Could you check a few things on this model? Use its own coordinates, in mm. Face numbers are marked on the shaded views. A direction names the side the tool comes from. Give positions to 0.01 mm unless a question says otherwise; leave off trailing zeros. Write each loop counter-clockwise with the first axis right and the second up, starting at its lowest first coordinate (ties: lowest second). Pieces come first, ordered by that corner, then holes. Notation, with made-up numbers: (6.5, 55.25) -> (34.5, 55.25) arc R26 ccw to (34.5, 73.25) -> close; hole circle Ø3 at (53, 21.5). An arc over 180 degrees is marked (long way). One line per question, with ' | ' between items.
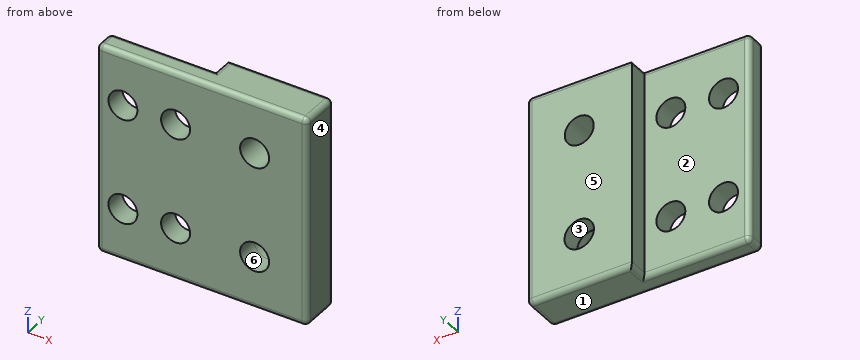
Autodesk Inventor part; units mm, degrees
ref_plane "YZ Plane" through (0, 0, 0) normal (1, 0, 0) x (0, 1, 0)
ref_plane "XZ Plane" through (0, 0, 0) normal (0, 1, 0) x (-1, 0, 0)
ref_plane "XY Plane" through (0, 0, 0) normal (0, 0, 1) x (1, 0, 0)
sketch "Sketch1" plane through (0, 0, 0) normal (0, 1, 0) x (-1, 0, 0)
  line L0 (17.7143, 25.1429) -> (-22.2857, 25.1429)
  line L1 (-22.2857, 25.1429) -> (-22.2857, -14.8571)
  line L2 (-22.2857, -14.8571) -> (17.7143, -14.8571)
  line L3 (17.7143, -14.8571) -> (17.7143, 25.1429)
  circle A0 centre (12.7143, 15.1429) radius 2.75
  circle A1 centre (12.7143, -4.8571) radius 2.75
  circle A2 centre (2.7143, -4.8571) radius 2.75
  circle A3 centre (2.7143, 15.1429) radius 2.75
  circle A4 centre (-12.2857, 15.1429) radius 2.75
  circle A5 centre (-12.2857, -4.8571) radius 2.75
  point P0 (0, 0)
  dimension "d1" = 40
  dimension "d2" = 5.5
  dimension "d3" = 5.5
  dimension "d4" = 5.5
  dimension "d5" = 5.5
  dimension "d6" = 5.5
  dimension "d7" = 5.5
  dimension "d9" = 10
  dimension "d12" = 20
  dimension "d13" = 10
  dimension "d17" = 5
  dimension "d28" = 10
  dimension "d32" = 15
extrude "Extrusion1" add sketch "Sketch1" along normal blind 4
sketch "Sketch2" plane through (0, 4, 0) normal (0, 1, 0) x (1, 0, 0)
  line L0 (22.2857, -25.1429) -> (22.2857, 14.8571)
  line L1 (22.2857, 14.8571) -> (2.2857, 14.8571)
  line L2 (2.2857, 14.8571) -> (2.2857, -25.1429)
  line L3 (2.2857, -25.1429) -> (22.2857, -25.1429)
  line L4 (22.2857, -25.1429) -> (22.2857, 14.8571)
  point P0 (0, 0)
  dimension "d30" = 20
  dimension "d31" = 40
extrude "Extrusion2" add sketch "Sketch2" along normal blind 3.7
sketch "Sketch3" plane through (12.2857, 4, -4.8571) normal (0, -1, 0) x (1, 0, 0)
  circle A0 centre (0, 0) radius 2.7975
  circle A1 centre (0, 20) radius 2.75
  line L0 (10, -10) -> (-30, -10)
  line L1 (10, 30) -> (10, -10)
  point P0 (-12.2857, 4.8571)
  dimension "d21" = 20
  dimension "d22" = 5.5
  dimension "d23" = 10
  dimension "d24" = 10
extrude "Extrusion3" cut sketch "Sketch3" against normal blind 3.7
fillet "Fillet2" radius 1 16 edges at (2.2857, 0, 25.1429) (-7.7143, 4, 25.1429) (12.2857, 7.7, 25.1429) (22.2857, 3.85, 25.1429) (22.2857, 7.7, 5.1429) (12.2857, 7.7, -14.8571) (-17.7143, 4, 5.1429) (-7.7143, 4, -14.8571) (2.2857, 0, -14.8571) (-17.7143, 2, -14.8571) (-17.7143, 0, 5.1429) (-17.7143, 2, 25.1429) (22.2857, 3.85, -14.8571) (22.2857, 0, 5.1429) (2.2857, 5.85, 25.1429) (2.2857, 5.85, -14.8571)
properties part number "syringepumpplate"
Q1. Imagine slicing it at A-A on x = -12.5. Please give me the cut outline in (y, z).
Answer below:
outline: (0, -13.86) arc R1 ccw to (1, -14.86) -> (3, -14.86) arc R1 ccw to (4, -13.86) -> (4, -7.6) -> (0, -7.6) -> close; (0, -2.12) -> (4, -2.12) -> (4, 12.4) -> (0, 12.4) -> close; (0, 17.88) -> (4, 17.88) -> (4, 24.14) arc R1 ccw to (3, 25.14) -> (1, 25.14) arc R1 ccw to (0, 24.14) -> close
Q2. Imagine slicing it at B-B on y = 5. Count the separate pieces of the cut face and the enclosed holes in it, and give its area (3 significant figures).
Answer below:
separate pieces: 1 | enclosed holes: 2 | area: 751 mm^2
Q3. If we mould it in two halves opening along X, with no side actions, what happens to the marked faces 4, 5 and 6? For each: +X half, -X half, draft (parallel to the pull), parting line (faces both ways), or undercut.
Answer below:
face 4: +X half | face 5: draft | face 6: undercut
Q4. On a 3-axis mill with a long thin cutter (end or side, diameter ignored), from which of +Z, -Z, +X, -X, +Y, -Y can I reach the whole of each face in a straight line? I mean the marked faces 1, 2 and 3. Say none if no direction works.
Answer below:
face 1: -Z, +X, -X, +Y, -Y | face 2: +Z, -Z, -X, +Y | face 3: +Y
Q5. Imagine slicing it at D-D on y = 1.5. Please give me the cut outline in (x, z), and give its area (3 significant figures).
Answer below:
outline: (-17.71, -13.86) arc R1 ccw to (-16.71, -14.86) -> (21.29, -14.86) arc R1 ccw to (22.29, -13.86) -> (22.29, 24.14) arc R1 ccw to (21.29, 25.14) -> (-16.71, 25.14) arc R1 ccw to (-17.71, 24.14) -> close; hole circle Ø5.5 at (-12.71, -4.86); hole circle Ø5.5 at (-12.71, 15.14); hole circle Ø5.5 at (-2.71, -4.86); hole circle Ø5.5 at (-2.71, 15.14); hole circle Ø5.5 at (12.29, -4.86); hole circle Ø5.5 at (12.29, 15.14) | area: 1,460 mm^2
Q6. Imagine slicing it at C-C on z = 20. Please give me the cut outline in (x, y), and give its area (3 significant figures).
Answer below:
outline: (-17.71, 1) arc R1 ccw to (-16.71, 0) -> (21.29, 0) arc R1 ccw to (22.29, 1) -> (22.29, 6.7) arc R1 ccw to (21.29, 7.7) -> (2.29, 7.7) -> (2.29, 4) -> (-16.71, 4) arc R1 ccw to (-17.71, 3) -> close | area: 233 mm^2
Q7. If I drill on line 1 along X through (y, z) = (3, -5); line 2 along X through (y, z) = (0.5, 17); line 3 along Z through (x, y) = (14, 6.25), over which ranges is the centre line in solid material (lowest first)?
Answer below:
line 1: x = -17.71 to -15.46, -9.97 to -5.46, 0.03 to 9.54, 15.03 to 22.29 | line 2: x = -17.58 to -14.74, -10.69 to -4.74, -0.69 to 10.26, 14.31 to 22.15 | line 3: z = -14.86 to -7.07, -2.65 to 12.99, 17.29 to 25.14
Q8. Will these pins go through, and if not, where does the flat tip stop? pin 1 (4.5 mm diameter, centred on x = 12.29, z = 15.14, fed in from +Y); pin 2 (4.5 mm diameter, centred on x = 11, z = -3.5, fed in from +Y); pin 3 (9.5 mm diameter, centred on x = -6, z = 10, fed in from +Y); pin 4 (1.1 mm diameter, centred on y = 6, z = 14.5, fed in from -X).
Answer below:
pin 1: passes through | pin 2: stops at y = 7.7 | pin 3: stops at y = 4 | pin 4: stops at x = 2.29
